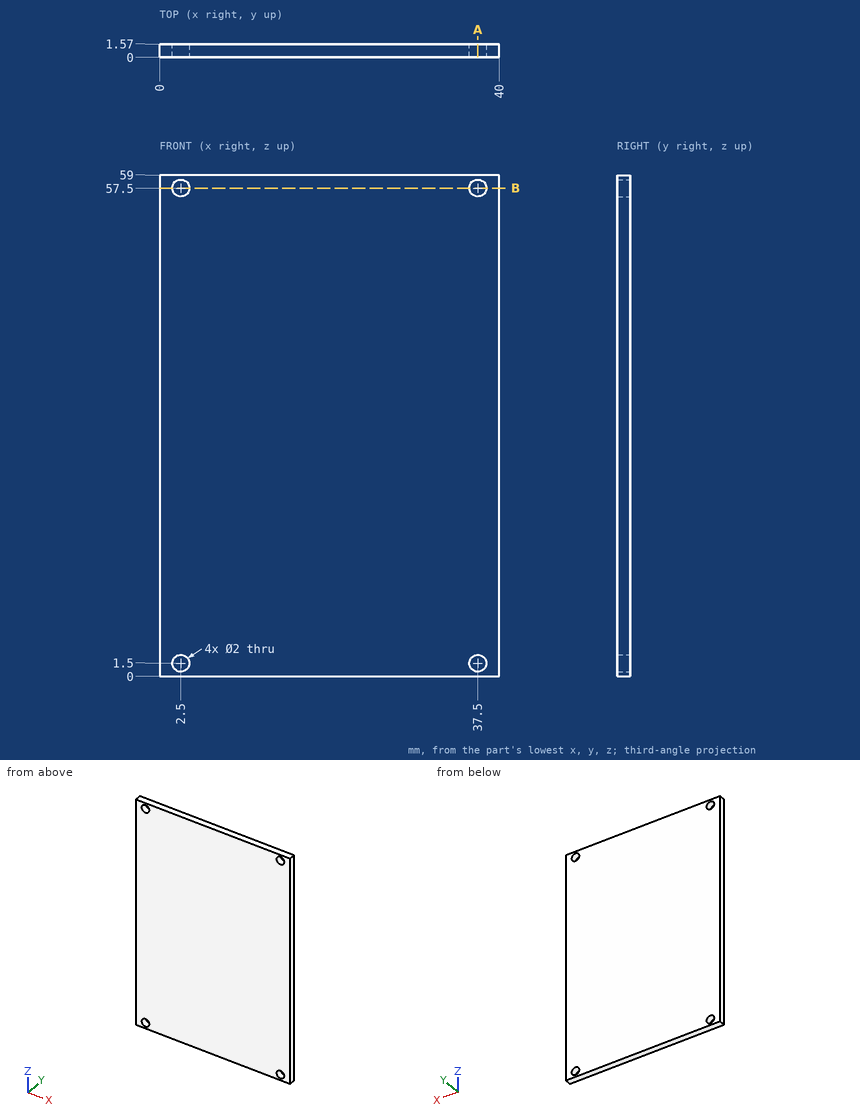
Input: dimensioned drawing with shaded views. Units: mm. Origin: part minimum x, y, z. Coordinates: 2 decimals unless noted, no trailing zeros. Loops run counter-clockwise (first coordinate to the right, second up) from the corner with the lowest first, then second, coordinate; pieces in that order, holes last. Notation, with made-up numbers: (-19.5, 79) -> (-8.5, 79) arc R25 ccw to (-8.5, 92) -> close; hole circle Ø11 at (18.25, 26). An arc over 180 degrees is marked (long way). One line per item, written item: value. Start each with the question number.
Q1. Contact query for flat-ended pins moving along their axis: P1, Ø2.5, axis at x = 2.5, z = 57.5, coming from the -Y side; P2, Ø1.2, axis at x = 37.5, z = 57.5, coming from the -Y side. Output: stop coordinate, or through.
Q2. Section query A-A, the plane x = 37.5. Return the cut outline in (y, z).
Q3. Line query: line 1 along X through (y, z) = (1.2, 1.5); line 2 along Z through (x, y) = (2.5, 0.85). Output: solid intervals per line, ascending.
Q4. Section query B-B, the plane z = 57.5. Return the cut outline in (x, y), and give its area (3 significant figures).
Results:
1. P1: y = 0
1. P2: through
2. outline: (0, 0) -> (1.57, 0) -> (1.57, 0.5) -> (0, 0.5) -> close; (0, 2.5) -> (1.57, 2.5) -> (1.57, 56.5) -> (0, 56.5) -> close; (0, 58.5) -> (1.57, 58.5) -> (1.57, 59) -> (0, 59) -> close
3. line 1: 0 to 1.5, 3.5 to 36.5, 38.5 to 40
3. line 2: 0 to 0.5, 2.5 to 56.5, 58.5 to 59
4. outline: (0, 0) -> (1.5, 0) -> (1.5, 1.57) -> (0, 1.57) -> close; (3.5, 0) -> (36.5, 0) -> (36.5, 1.57) -> (3.5, 1.57) -> close; (38.5, 0) -> (40, 0) -> (40, 1.57) -> (38.5, 1.57) -> close
4. area: 56.5 mm^2
